Design review of the part built by this model. Coordinates are the model's own, in mm. Face numbers are marked on the shaded views. A direction names the side the tool comes from. Give positions to 0.01 mm unless a question says otherwise; leave off trailing zeros. Order: outer loops, then holes, each group sorted by start corner. A loop starts at its lowest first (then second) coordinate and runs counter-clockwise, first axis right, second up. Notation, with made-up numbers: (36, -10) -> (72, -10) arc R31 ccw to (72, 21) -> close; hole circle Ø10 at (-10, 60). An arc over 180 degrees is marked (long way). One line per item, written item: value.
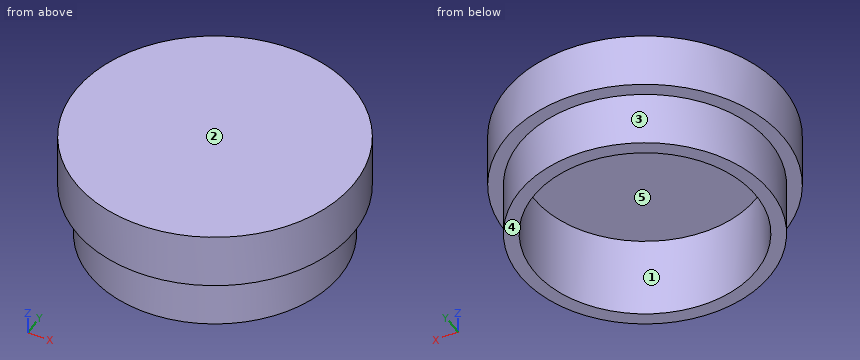
from build123d import *

# Parameters (mm, degrees)
SKETCH_R      = 25
PAD_DEPTH     = 10
SKETCH001_R   = 22.5
SKETCH001_R_2 = 20
PAD001_DEPTH  = 10
SKETCH002_R   = 20
POCKET_DEPTH  = 5


with BuildPart() as part:
    # Sketch → Pad (new body)
    with BuildSketch(Plane.XY):
        Circle(SKETCH_R)
    extrude(amount=PAD_DEPTH)

    # Sketch001 (on Face2 of Pad) → Pad001 (join)
    with BuildSketch(Plane(origin=(0, 0, 0), x_dir=(1, 0, 0), z_dir=(0, 0, -1))):
        Circle(SKETCH001_R)
        Circle(SKETCH001_R_2, mode=Mode.SUBTRACT)
    extrude(amount=PAD001_DEPTH)

    # Sketch002 (on Face7 of Pad001) → Pocket (cut)
    with BuildSketch(Plane(origin=(0, 0, 0), x_dir=(1, 0, 0), z_dir=(0, 0, -1))):
        Circle(SKETCH002_R)
    extrude(amount=-POCKET_DEPTH, mode=Mode.SUBTRACT)


solid = part.part
Item 1: Add section C-C on z = 1.25. Give the boundary of the cut face in (x, y), plus the area to 3 significant figures.
Returned:
outline: circle Ø50 at (0, 0); hole circle Ø40 at (0, 0)
area: 707 mm²
Item 2: Add section D-D on z = 8. Give the boundary of the cut face in (x, y).
Returned:
outline: circle Ø50 at (0, 0)
Item 3: Clearance check with flat-ended pins moving along their axes: P1, Ø1.5, axis at x = -1.5, z = -2, coming from the +Y side; P2, Ø1, axis at y = 4, z = -4, coming from the -X side; P3, Ø3, axis at x = -18.5, z = 2, coming from the -Y side. State where each tip first meets the part, or that it passes through.
Returned:
P1: y = 22.49
P2: x = -22.23
P3: y = -18.33
Item 4: Draft analysis for pull direction Y (two halves, no side actions). For the marked faces 1, 2 and 3, state which applies: pulls with the +Y half, pulls with the -Y half, needs draft (parallel to the pull), parting line crosses it, or undercut.
Returned:
face 1: undercut
face 2: needs draft
face 3: parting line crosses it
Item 5: Add section B-B on x = 12. Give the boundary of the cut face in (y, z), plus the area to 3 significant figures.
Returned:
outline: (-21.93, 0) -> (-19.03, 0) -> (-19.03, -10) -> (-16, -10) -> (-16, 5) -> (16, 5) -> (16, -10) -> (19.03, -10) -> (19.03, 0) -> (21.93, 0) -> (21.93, 10) -> (-21.93, 10) -> close
area: 339 mm²
Item 6: To check wall thickness, follow line 1 along X through (y, z) = (0, -7); line 2 along Z through (x, y) = (18, 7). State the ranges of each line that lie inside material, in increasing order. Write a range as from..to.
Returned:
line 1: -22.5..-20, 20..22.5
line 2: 5..10
Item 7: Add section A-A on y = 0. Give the boundary of the cut face in (x, z).
Returned:
outline: (-25, 0) -> (-22.5, 0) -> (-22.5, -10) -> (-20, -10) -> (-20, 5) -> (20, 5) -> (20, -10) -> (22.5, -10) -> (22.5, 0) -> (25, 0) -> (25, 10) -> (-25, 10) -> close
Item 8: Machinability: for the marked faces 4 and 5, which of the approach directions +Z, -Z, +X, -X, +Y, -Y give a long, thin tool a straight path to every point of the face, cutting with its end or side? Answer none if there is none.
Returned:
face 4: -Z, +X, -X, +Y, -Y
face 5: -Z
